```python
from build123d import *

# Parameters (mm, degrees)
BOSS_EXTRUDE1_DEPTH = 400
SKETCH2_R           = 1.5
CUT_EXTRUDE1_DEPTH  = 10
LPATTERN1_COUNT     = 16
LPATTERN1_PITCH     = 25


with BuildPart() as part:
    # Sketch1 → Boss-Extrude1 (new body)
    with BuildSketch(Plane.XY):
        Polygon((-6, -2.75), (-6, -4), (6, -4), (6, -2.75), (5.25, -2), (4, -2), (4, -1), (5.25, -1), (6, -0.25), (6, 4), (-3.888196601, 4), (-4, 3.9), (-4.111803399, 4), (-6, 4), (-6, -0.25), (-5.25, -1), (-4, -1), (-4, -2), (-5.25, -2), align=None)
    extrude(amount=BOSS_EXTRUDE1_DEPTH)

    # Sketch2 → Cut-Extrude1 (cut)
    with BuildSketch(Plane.XZ.offset(4)):
        with Locations(Location((0, 12.5, 0), (0, 0, 270))):
            Circle(SKETCH2_R)
    cut_extrude1 = extrude(amount=-CUT_EXTRUDE1_DEPTH, mode=Mode.SUBTRACT)

    # LPattern1: Cut-Extrude1 ×16
    with Locations(*[(0, 0, i * LPATTERN1_PITCH) for i in range(1, LPATTERN1_COUNT)]):
        add(cut_extrude1, mode=Mode.SUBTRACT)


solid = part.part
```
Model file for the job. Use its own axes, mm. Round coordinates to 2 decimals unless told otherwise and drop trailing zeros. Loops run counter-clockwise (first coordinate to the right, second up) from the corner with the lowest first, then second, coordinate; pieces in that order, holes last. Notation, with made-up numbers: M -28.75,87.5 L -6.75,87.5 A18 ccw -6.75,93.5 Z; hole C 67.5,11 d2. An arc over 180 degrees is marked long. Put each result on its own line as item: value. Start each with the question number.
Item 1: Cut at A-A (z = 244). List the corners of the cut face in (x, y), then the cut area to 3 significant figures.
Item 2: Drill centre lines: line 1 along X through (y, z) = (0, 287.5); line 2 along Y through (x, z) = (5.25, 163); line 3 along X through (y, z) = (-1.25, 254). Where is each one in solid material? Low to high.
Item 3: Mould opens along Y. For faces 1 (the face through (0, -4, 197)), 2 (the face through (0, 0, 400)), 3 (the face through (1, 4, 197)) say: released by +Y, released by -Y, zero draft, split by the parting line, or undercut.
Answer block:
1. outline: M -6,-4 L 6,-4 L 6,-2.75 L 5.25,-2 L 4,-2 L 4,-1 L 5.25,-1 L 6,-0.25 L 6,4 L -3.89,4 L -4,3.9 L -4.11,4 L -6,4 L -6,-0.25 L -5.25,-1 L -4,-1 L -4,-2 L -5.25,-2 L -6,-2.75 Z
1. area: 90.9 mm2
2. line 1: -6 to -1.5, 1.5 to 6
2. line 2: -4 to -2, -1 to 4
2. line 3: -4 to 4
3. face 1: released by -Y
3. face 2: zero draft
3. face 3: released by +Y
